Design review of the part built by this model. Coordinates are the model's own, in mm. A direction names the side the tool comes from. Coordinates: 2 decimals unless noted, no trailing zeros. Loops run counter-clockwise (first coordinate to the right, second up) from the corner with the lowest first, then second, coordinate; pieces in that order, holes last. Notation, with made-up numbers: M 67,51.5 L 86,51.5 A23 cw 86,84.5 Z; hole C 77.25,20 d5. An arc over 180 degrees is marked long. One line per item, written item: value.
```python
from build123d import *

# Parameters (mm, degrees)
SALIENTE_EXTRUIR1_DEPTH = 5.1


with BuildPart() as part:
    # Croquis1 → Saliente-Extruir1 (new body)
    with BuildSketch(Plane.XY):
        with BuildLine():
            Line((0, 0), (10, 0))
            Line((10, 0), (10, 8.8))
            Line((10, 8.8), (14.8, 8.8))
            Line((14.8, 8.8), (14.8, 0))
            Line((14.8, 0), (24.8, 0))
            Line((24.8, 0), (24.8, 13.6))
            ThreePointArc((24.8, 13.6), (25.971572875, 16.428427125), (28.8, 17.6))
            Line((28.8, 17.6), (42.4, 17.6))
            Line((42.4, 17.6), (42.4, 27.6))
            Line((42.4, 27.6), (33.6, 27.6))
            Line((33.6, 27.6), (33.6, 32.4))
            Line((33.6, 32.4), (42.4, 32.4))
            Line((42.4, 32.4), (42.4, 42.4))
            Line((42.4, 42.4), (28.8, 42.4))
            ThreePointArc((28.8, 42.4), (25.971572875, 43.571572875), (24.8, 46.4))
            Line((24.8, 46.4), (24.8, 60))
            Line((24.8, 60), (14.8, 60))
            Line((14.8, 60), (14.8, 51.2))
            Line((14.8, 51.2), (10, 51.2))
            Line((10, 51.2), (10, 60))
            Line((10, 60), (0, 60))
            Line((0, 60), (0, 46.4))
            ThreePointArc((0, 46.4), (-1.171572875, 43.571572875), (-4, 42.4))
            Line((-4, 42.4), (-17.6, 42.4))
            Line((-17.6, 42.4), (-17.6, 32.4))
            Line((-17.6, 32.4), (-8.8, 32.4))
            Line((-8.8, 32.4), (-8.8, 27.6))
            Line((-8.8, 27.6), (-17.6, 27.6))
            Line((-17.6, 27.6), (-17.6, 17.6))
            Line((-17.6, 17.6), (-4, 17.6))
            ThreePointArc((-4, 17.6), (-1.171572875, 16.428427125), (0, 13.6))
            Line((0, 13.6), (0, 0))
        make_face()
    extrude(amount=SALIENTE_EXTRUIR1_DEPTH)


solid = part.part
```
(1) To check wall thickness, follow line 1 along X through (y, z) = (57, 3.1); line 2 along Y through (x, z) = (34.5, 0.75); line 3 along Y through (x, z) = (14.5, 2.4). State the ranges of each line that lie inside material, in increasing order. Write a range as [from, to].
Reply:
line 1: x = [0, 10], [14.8, 24.8]
line 2: y = [17.6, 27.6], [32.4, 42.4]
line 3: y = [8.8, 51.2]
(2) Mouldability with a two-part tool opening along Y and no side actions: class faces 6 (the flat face through (0, 53, 3)), 7 (the cylindrical face through (25.941, 16.397, 2.514)), 8 (the flat face through (-8.8, 30, 3)) as released by +Y, released by -Y, zero draft, split by the parting line, or undercut.
Reply:
face 6: zero draft
face 7: released by -Y
face 8: undercut
(3) Insertion check: pin 1 (2.5 mm diameter, centred on x = 39, z = 3, fed in from +Y); pin 2 (1 mm diameter, centred on x = 16.5, z = 1.5, fed in from -Y); pin 3 (1.4 mm diameter, centred on y = 31, z = 3, fed in from -X); pin 4 (2.5 mm diameter, centred on x = 33, z = 1.5, fed in from -Y). Each pin has a flat end and moves straight along its axis. Give the tip position at first contact, or say it passes through.
Reply:
pin 1: stops at y = 42.4
pin 2: stops at y = 0
pin 3: stops at x = -8.8
pin 4: stops at y = 17.6
(4) We need section C-C on y = 29.5. State the section outline as (x, z) points, then the cut area to 3 significant figures.
Reply:
outline: M -8.8,0 L 33.6,0 L 33.6,5.1 L -8.8,5.1 Z
area: 216 mm2
(5) We need section D-D on x = -2.5. State the section outline as (y, z) points, then the cut area to 3 significant figures.
Reply:
outline: M 17.31,0 L 42.69,0 L 42.69,5.1 L 17.31,5.1 Z
area: 129 mm2
(6) We need section A-A on y = 5. State the section outline as (x, z) points, then the cut area to 3 significant figures.
Reply:
outline: M 0,0 L 10,0 L 10,5.1 L 0,5.1 Z; M 14.8,0 L 24.8,0 L 24.8,5.1 L 14.8,5.1 Z
area: 102 mm2
(7) Tool access review of faces 1 (the flat face through (14.8, 56, 3)), 2 (the flat face through (-11, 42.4, 3)), 3 (the flat face through (10, 4, 3)), 4 (the flat face through (24.8, 7, 3)), 5 (the flat face through (0, 7, 3)): name each direction out of +Z, -Z, +X, -X, +Y, -Y from which nothing blocks a thin tool from reaching the whole face with its end or side.
Reply:
face 1: +Z, -Z, +Y
face 2: +Z, -Z, -X, +Y
face 3: +Z, -Z, -Y
face 4: +Z, -Z, +X, -Y
face 5: +Z, -Z, -X, -Y
